Verification items for the finished model (mm, model axes). A direction names the side the tool comes from. Coordinates: 2 decimals unless noted, no trailing zeros. Loops run counter-clockwise (first coordinate to the right, second up) from the corner with the lowest first, then second, coordinate; pieces in that order, holes last. Notation, with made-up numbers: (74.5, -31.5) -> (96.5, -31.5) arc R36 cw to (96.5, 5.5) -> close; hole circle Ø5 at (-25.75, -9). An arc over 180 degrees is marked (long way). Answer as a JSON object with one key per item and string values. Group by question number.
Q1. Cross-section at A-A on z = 15. Record the boundary of the cut face in (x, y).
Q2. Cross-section at B-B on x = 44. Record the boundary of the cut face in (y, z).
Q3. Cross-section at C-C on z = 23.5. Record the boundary of the cut face in (x, y), and give its area (3 significant figures).
Q4. Cross-section at D-D on y = -36.5. Record the boundary of the cut face in (x, z), and give its area (3 significant figures).
Q5. Release check for a two-part mould opening along X. For faces 1 (the flat face through (22.352, -31, 3)), 2 (the flat face through (42.672, -31, 3)), 3 (the flat face through (45, -5.08, 13)), 4 (the flat face through (32, -26, 17.78)) record: released by +X, released by -X, zero draft, split by the parting line, or undercut.
Q6. Scan lines: L1, parallel to Y at x = 48.5, z = 1.5; L2, parallel to X at y = -4, z = 1.75; L3, parallel to X at y = -14.5, z = 22.5. Record each from-to range of solid material in increasing order.
Q7. Set-up check for faces 5 (the flat face through (23.64, -28.89, 6.37)), 6 (the flat face through (41.42, -28.68, 6.33)), 7 (the flat face through (32, -17.78, 13)): record each of +Z, -Z, +X, -X, +Y, -Y from which the full face is reachable in a straight line by a thin tool's end or side.
Q8. Gauge pin test, flat ends, axial feed: pin 1 Ø4 at (y, z) = (-28.5, 23) entering from -X; pin 2 Ø12 at (x, y) = (47.5, -41.5) entering from +Z; pin 3 Ø3 at (x, y) = (48, -15) entering from -Z; pin 4 Ø5.5 at (y, z) = (-30, 22.5) entering from +X. Record the tip position at first contact, or that the pin passes through.
```python
from build123d import *

# Parameters (mm, degrees)
BOSS_EXTRUDE2_DEPTH = 25.4
BOSS_EXTRUDE3_DEPTH = 7.62
SKETCH6_R           = 10.16
BOSS_EXTRUDE5_DEPTH = 25.4
FILLET4_R           = 12.7
CHAMFER3_SIZE       = 2.54
SKETCH7_W           = 20.32
SKETCH7_H           = 15.24
BOSS_EXTRUDE6_DEPTH = 7.62
CHAMFER4_SIZE       = 2.54


with BuildPart() as part:
    # Sketch2 → Boss-Extrude2 (new body)
    with BuildSketch(Plane.XY):
        Polygon((0, 0), (26.162, 0), (26.162, -5.08), (13.462, -5.08), (13.462, -17.78), (51.562, -17.78), (51.562, -5.08), (38.862, -5.08), (38.862, 0), (65.024, 0), (65.024, -22.86), (0, -22.86), align=None)
    extrude(amount=BOSS_EXTRUDE2_DEPTH)

    # Sketch4 → Boss-Extrude3 (add)
    with BuildSketch(Plane.XY.offset(25.4)):
        Polygon((32.512, -22.86), (22.352, -22.86), (22.352, -38.1), (42.672, -38.1), (42.672, -22.86), align=None)
    extrude(amount=-BOSS_EXTRUDE3_DEPTH)

    # Sketch6 → Boss-Extrude5 (add)
    with BuildSketch(Plane.XY.offset(25.4)):
        with Locations((32.512, -38.1)):
            Circle(SKETCH6_R)
    extrude(amount=-BOSS_EXTRUDE5_DEPTH)

    # Fillet4
    # the kernel refuses this fillet: 12.7 mm, written as the material it takes off along each edge
    with BuildSketch(Plane(origin=(65.024, -22.86, -31.75), x_dir=(-1, 0, 0), z_dir=(0, 0, 1)), Plane(origin=(0, -22.86, -31.75), x_dir=(0, 1, 0), z_dir=(0, 0, 1)), Plane(origin=(0, 0, -31.75), x_dir=(1, 0, 0), z_dir=(0, 0, 1))) as fillet4_piece_1:
        with BuildLine():
            CenterArc((FILLET4_R, -FILLET4_R), FILLET4_R, 90, 90)
            Line((0, -FILLET4_R), (-FILLET4_R * 0.02, -FILLET4_R))
            Line((-FILLET4_R * 0.02, -FILLET4_R), (-FILLET4_R * 0.02, FILLET4_R * 0.02))
            Line((-FILLET4_R * 0.02, FILLET4_R * 0.02), (FILLET4_R, FILLET4_R * 0.02))
            Line((FILLET4_R, FILLET4_R * 0.02), (FILLET4_R, 0))
        make_face()
    extrude(amount=88.9, mode=Mode.SUBTRACT)
    with BuildSketch(Plane(origin=(26.162, 0, -25.4), x_dir=(-1, 0, 0), z_dir=(0, 0, 1))) as fillet4_piece_2:
        with BuildLine():
            CenterArc((10.16, 12.7), FILLET4_R, 216.869897646, 53.130102354)
            Line((0, 5.08), (-0.2032, 4.9276))
            ThreePointArc((-0.2032, 4.9276), (-0.254, 2.54), (-0.254, 0))
            Line((-0.254, 0), (0, -0.254))
            Line((0, -0.254), (10.16, -0.254))
            Line((10.16, -0.254), (10.16, 0))
        make_face()
    extrude(amount=76.2, mode=Mode.SUBTRACT)
    with BuildSketch(Plane(origin=(38.862, 0, -25.4), x_dir=(0, -1, 0), z_dir=(0, 0, 1))) as fillet4_piece_3:
        with BuildLine():
            CenterArc((12.7, 10.16), FILLET4_R, 180, 53.130102354)
            Line((0, 10.16), (-0.254, 10.16))
            Line((-0.254, 10.16), (-0.254, 0))
            Line((-0.254, 0), (0, -0.254))
            ThreePointArc((0, -0.254), (2.54, -0.254), (4.9276, -0.2032))
            Line((4.9276, -0.2032), (5.08, 0))
        make_face()
    extrude(amount=76.2, mode=Mode.SUBTRACT)
    with BuildSketch(Plane(origin=(65.024, 0, -31.75), x_dir=(-1, 0, 0), z_dir=(0, 0, 1))) as fillet4_piece_4:
        with BuildLine():
            CenterArc((FILLET4_R, FILLET4_R), FILLET4_R, 180, 90)
            Line((0, FILLET4_R), (-FILLET4_R * 0.02, FILLET4_R))
            Line((-FILLET4_R * 0.02, FILLET4_R), (-FILLET4_R * 0.02, -FILLET4_R * 0.02))
            Line((-FILLET4_R * 0.02, -FILLET4_R * 0.02), (FILLET4_R, -FILLET4_R * 0.02))
            Line((FILLET4_R, -FILLET4_R * 0.02), (FILLET4_R, 0))
        make_face()
    extrude(amount=88.9, mode=Mode.SUBTRACT)

    # Chamfer3
    # the kernel refuses this chamfer: 2.54 mm, written as the material it takes off along each edge
    with BuildSketch(Plane(origin=(42.672, -44.632074789, 17.78), x_dir=(0.027495876610587302, 0, 0.9996219169112966), z_dir=(0, 1, 0))) as chamfer3_piece_1_section:
        Polygon((CHAMFER3_SIZE * 0.999621916911, -CHAMFER3_SIZE * 0.0274958766106), (-CHAMFER3_SIZE * 0.0274958766106, -CHAMFER3_SIZE * 0.999621916911), (0, 0), align=None)
    chamfer3_piece_1 = extrude(amount=21.772074789, mode=Mode.PRIVATE)
    chamfer3_piece_1 = chamfer3_piece_1 - Plane(origin=(32.512, -38.1, 18.664342035), x_dir=(1, 0, 0), z_dir=(0, 0, 1)) * Cylinder(10.16, 54, mode=Mode.PRIVATE)
    add(chamfer3_piece_1, mode=Mode.SUBTRACT)
    with BuildSketch(Plane(origin=(22.352, -22.86, 17.78), x_dir=(-0.02749587661058595, 0, 0.9996219169112968), z_dir=(0, -1, 0))) as chamfer3_piece_2_section:
        Polygon((CHAMFER3_SIZE * 0.999621916911, -CHAMFER3_SIZE * 0.0274958766106), (-CHAMFER3_SIZE * 0.0274958766106, -CHAMFER3_SIZE * 0.999621916911), (0, 0), align=None)
    chamfer3_piece_2 = extrude(amount=21.772074789, mode=Mode.PRIVATE)
    chamfer3_piece_2 = chamfer3_piece_2 - Plane(origin=(32.512, -38.1, 18.664342036), x_dir=(1, 0, 0), z_dir=(0, 0, 1)) * Cylinder(10.16, 54, mode=Mode.PRIVATE)
    add(chamfer3_piece_2, mode=Mode.SUBTRACT)

    # Sketch7 → Boss-Extrude6 (add)
    with BuildSketch(Plane(origin=(0, 0, 0), x_dir=(-1, 0, 0), z_dir=(0, 0, -1))):
        with Locations((-32.512, -30.48)):
            Rectangle(SKETCH7_W, SKETCH7_H)
    extrude(amount=-BOSS_EXTRUDE6_DEPTH)

    # Chamfer4
    # the kernel refuses this chamfer: 2.54 mm, written as the material it takes off along each edge
    with BuildSketch(Plane(origin=(22.352, -44.632074789, 7.62), x_dir=(0.9996219169112966, 0, 0.027495876610586282), z_dir=(0, 1, 0))) as chamfer4_piece_1_section:
        Polygon((CHAMFER4_SIZE * 0.999621916911, CHAMFER4_SIZE * 0.0274958766106), (-CHAMFER4_SIZE * 0.0274958766106, CHAMFER4_SIZE * 0.999621916911), (0, 0), align=None)
    chamfer4_piece_1 = extrude(amount=21.772074789, mode=Mode.PRIVATE)
    chamfer4_piece_1 = chamfer4_piece_1 - Plane(origin=(32.512, -38.1, 6.735657964), x_dir=(1, 0, 0), z_dir=(0, 0, 1)) * Cylinder(10.16, 54, mode=Mode.PRIVATE)
    add(chamfer4_piece_1, mode=Mode.SUBTRACT)
    with BuildSketch(Plane(origin=(42.672, -22.86, 7.62), x_dir=(0.027495876610587288, 0, -0.9996219169112968), z_dir=(0, -1, 0))) as chamfer4_piece_2_section:
        Polygon((CHAMFER4_SIZE * 0.999621916911, -CHAMFER4_SIZE * 0.0274958766106), (-CHAMFER4_SIZE * 0.0274958766106, -CHAMFER4_SIZE * 0.999621916911), (0, 0), align=None)
    chamfer4_piece_2 = extrude(amount=21.772074789, mode=Mode.PRIVATE)
    chamfer4_piece_2 = chamfer4_piece_2 - Plane(origin=(32.512, -38.1, 6.735657965), x_dir=(1, 0, 0), z_dir=(0, 0, 1)) * Cylinder(10.16, 54, mode=Mode.PRIVATE)
    add(chamfer4_piece_2, mode=Mode.SUBTRACT)


solid = part.part
```
Computed values:
{
 "1": {"outline": "(0.06, -11.43) arc R12.7 ccw to (12.7, -22.86) -> (52.32, -22.86) arc R12.7 ccw to (64.96, -11.43) arc R12.7 ccw to (52.32, 0) -> (49.02, 0) arc R12.7 ccw to (38.86, -5.08) -> (51.56, -5.08) -> (51.56, -17.78) -> (13.46, -17.78) -> (13.46, -5.08) -> (26.16, -5.08) arc R12.7 ccw to (16, 0) -> (12.7, 0) arc R12.7 ccw to start; circle Ø20.32 at (32.51, -38.1)"},
 "2": {"outline": "(-22.86, 0) -> (-17.78, 0) -> (-17.78, 25.4) -> (-22.86, 25.4) -> close; (-5.08, 0) -> (-1.04, 0) -> (-1.04, 25.4) -> (-5.08, 25.4) -> close"},
 "3": {"outline": "(0.06, -11.43) arc R12.7 ccw to (12.7, -22.86) -> (22.35, -22.86) -> (22.35, -38.1) arc R10.16 ccw to (42.67, -38.1) -> (42.67, -22.86) -> (52.32, -22.86) arc R12.7 ccw to (64.96, -11.43) arc R12.7 ccw to (52.32, 0) -> (49.02, 0) arc R12.7 ccw to (38.86, -5.08) -> (51.56, -5.08) -> (51.56, -17.78) -> (13.46, -17.78) -> (13.46, -5.08) -> (26.16, -5.08) arc R12.7 ccw to (16, 0) -> (12.7, 0) arc R12.7 ccw to start", "area": "1,240 mm²"},
 "4": {"outline": "(22.35, 0) -> (42.67, 0) -> (42.67, 5.08) -> (42.55, 5.21) -> (42.55, 20.19) -> (42.67, 20.32) -> (42.67, 25.4) -> (22.35, 25.4) -> (22.35, 20.32) -> (22.48, 20.19) -> (22.48, 5.21) -> (22.35, 5.08) -> close", "area": "512 mm²"},
 "5": {"face 1": "released by -X", "face 2": "released by +X", "face 3": "undercut", "face 4": "zero draft"},
 "6": {"L1": "y = -22.86 to -17.78, -5.08 to -0.01", "L2": "x = 3.45 to 25.25, 39.77 to 61.58", "L3": "x = 0.76 to 13.46, 51.56 to 64.26"},
 "7": {"face 5": "-X", "face 6": "+X", "face 7": "+Z, -Z"},
 "8": {"pin 1": "stops at x = 22.35", "pin 2": "stops at z = 25.4", "pin 3": "passes through", "pin 4": "stops at x = 42.67"}
}
